from build123d import *

# Parameters (mm, degrees)
ESQUISSE1_R                  = 5
BOSS_EXTRU_1_DEPTH           = 12
ESQUISSE2_R                  = 5
BOSS_EXTRU_2_DEPTH           = 2
ESQUISSE3_R                  = 1.5
ENL_V_MAT_EXTRU_1_DEPTH      = 14
R_P_TITION_CIRCULAIRE1_COUNT = 8


with BuildPart() as part:
    # Esquisse1 → Boss.-Extru.1 (new body)
    with BuildSketch(Plane(origin=(0, 0, 0), x_dir=(1, 0, 0), z_dir=(0, 1, 0))):
        with Locations(Location((0, 0, 0), (0, 0, 270))):
            Circle(ESQUISSE1_R)
        with BuildLine():
            Line((2.236067977, -2), (-2.236067977, -2))
            ThreePointArc((-2.236067977, -2), (0, 3), (2.236067977, -2))
        make_face(mode=Mode.SUBTRACT)
    extrude(amount=BOSS_EXTRU_1_DEPTH)

    # Esquisse2 → Boss.-Extru.2 (add)
    with BuildSketch(Plane(origin=(0, 12, 0), x_dir=(1, 0, 0), z_dir=(0, 1, 0))):
        with Locations(Location((0, 0, 0), (0, 0, 270))):
            Circle(ESQUISSE2_R)
    extrude(amount=BOSS_EXTRU_2_DEPTH)

    # Esquisse3 → Enlèv. mat.-Extru.1 (cut)
    with BuildSketch(Plane(origin=(0, 14, 0), x_dir=(1, 0, 0), z_dir=(0, 1, 0))):
        with Locations((0, 5.5)):
            Circle(ESQUISSE3_R)
    enl_v_mat_extru_1 = extrude(amount=-ENL_V_MAT_EXTRU_1_DEPTH, mode=Mode.SUBTRACT)

    # Répétition circulaire1: Enlèv. mat.-Extru.1 ×8 about axis
    r_p_tition_circulaire1_axis = Axis((0, 0, 0), (0, 1, 0))
    for i in range(1, R_P_TITION_CIRCULAIRE1_COUNT):
        add(enl_v_mat_extru_1.rotate(r_p_tition_circulaire1_axis, i * 360 / R_P_TITION_CIRCULAIRE1_COUNT), mode=Mode.SUBTRACT)


solid = part.part
Geometry check sheet. Reference: the model listing, model coordinates, mm. A direction names the side the tool comes from. Round coordinates to 2 decimals unless told otherwise and drop trailing zeros. Order: outer loops, then holes, each group sorted by start corner. A loop starts at its lowest first (then second) coordinate and runs counter-clockwise, first axis right, second up. Notation, with made-up numbers: (11.25, 14.25) - (53.25, 14.25) arc R17 cw to (53.25, 25.25) - close; hole circle Ø5 at (-33.75, -36.75). An arc over 180 degrees is marked (long way). One line per question, with ' | ' between items. Start each with the question number.
(1) Sectioned sample at B-B on x = 0. Record the cut outline in (y, z), and give its area (3 significant figures).
(2) Thickness scan on L1, parallel to Y at x = 2, z = -0.25; L2, parallel to Z at x = 0.5, y = 9.25; L3, parallel to Z at x = 1.25, y = 0.5. Record the ranges inside material, lowest first. Write a range as [from, to].
(3) Depth check by flat-ended pin: pin 1 Ø1.5 at (x, y) = (-3, 7.5) entering from -Z; pin 2 Ø3 at (x, y) = (3.5, 4.5) entering from -Z; pin 3 Ø1.5 at (x, y) = (-0.5, 7.5) entering from -Z. Enter the tip coordinate at first touch or a pass-through.
(4) Sectioned sample at D-D on z = -3.75. Record the cut outline in (x, y), and give its area (3 significant figures).
(5) Sectioned sample at C-C on z = 0. Record the cut outline in (x, y), and give its area (3 significant figures).
(6) Release check for a two-part mould opening along Z. For faces 3 (the cylindrical face through (0, 7, 4)), 4 (the cylindrical face through (4, 7, 0)), 5 (the cylindrical face through (4.62, 6.9, -1.91)) record: released by +Z, released by -Z, zero draft, split by the parting line, or undercut.
(7) Sectioned sample at A-A on y = 8.75. Record the cut outline in (x, z), and give its area (3 significant figures).
(8) Access from +Z, -Z, +X, -X, +Y, -Y to the whole of each face (thin tool, end or side, straight path). Record for faces 1 (the cylindrical face through (-1.921, 6.902, 4.616)), 2 (the flat face through (0, 12, -1)).
Conclusion:
1) outline: (0, -4) - (14, -4) - (14, 4) - (0, 4) - (0, 2) - (12, 2) - (12, -3) - (0, -3) - close | area: 52.0 mm2
2) L1: y = [12, 14] | L2: z = [-4.09, -2.96], [2, 4.09] | L3: z = [-4.67, -2.73], [2, 4.67]
3) pin 1: stops at z = -4.47 | pin 2: stops at z = -4.58 | pin 3: stops at z = -4.67
4) outline: (-2.4, 0) - (2.4, 0) - (2.4, 14) - (-2.4, 14) - close | area: 67.1 mm2
5) outline: (-4, 0) - (-3, 0) - (-3, 12) - (3, 12) - (3, 0) - (4, 0) - (4, 14) - (-4, 14) - close | area: 40.0 mm2
6) face 3: released by +Z | face 4: undercut | face 5: released by -Z
7) outline: (-4.82, -1.34) arc R5 ccw to (-4.35, -2.46) arc R1.5 cw to (-2.46, -4.35) arc R5 ccw to (-1.34, -4.82) arc R1.5 cw to (1.34, -4.82) arc R5 ccw to (2.46, -4.35) arc R1.5 cw to (4.35, -2.46) arc R5 ccw to (4.82, -1.34) arc R1.5 cw to (4.82, 1.34) arc R5 ccw to (4.35, 2.46) arc R1.5 cw to (2.46, 4.35) arc R5 ccw to (1.34, 4.82) arc R1.5 cw to (-1.34, 4.82) arc R5 ccw to (-2.46, 4.35) arc R1.5 cw to (-4.35, 2.46) arc R5 ccw to (-4.82, 1.34) arc R1.5 cw to start; hole (-2.24, 2) arc R3 ccw (long way) to (2.24, 2) - close | area: 38.3 mm2
8) face 1: +Z, -X, +Y, -Y | face 2: -Y
